Autodesk Inventor part; units mm, degrees
ref_plane "工作平面1" through (65, 2, 0) normal (-1, 0, 0) x (0, 0, 1)
ref_plane "YZ Plane" through (0, 0, 0) normal (1, 0, 0) x (0, 1, 0)
ref_plane "XZ Plane" through (0, 0, 0) normal (0, 1, 0) x (-1, 0, 0)
sketch "草圖1" plane through (0, 0, 0) normal (0, 0, 1) x (1, 0, 0)
  line L0 (0, 0) -> (-7.8042, 0) construction
  line L1 (0, 0) -> (0, -16.694) construction
  line L2 (0, 2) -> (0, 13)
  line L3 (310, 145) -> (310, 102)
  line L4 (130, 19.7875) -> (130, 13) construction
  line L5 (128, 0) -> (2, 0)
  line L6 (310, 145) -> (368, 145)
  line L7 (375, 138) -> (375, 109)
  line L8 (368, 102) -> (310, 102)
  line L9 (332, 127.5) -> (354, 127.5)
  arc A0 (354, 119.5) -> (354, 127.5) centre (354, 123.5) ccw
  line L10 (354, 119.5) -> (332, 119.5)
  arc A1 (332, 127.5) -> (332, 119.5) centre (332, 123.5) ccw
  arc A2 (10.0615, 42.1637) -> (0, 28) centre (15, 28) ccw
  line L11 (10.0615, 42.1637) -> (303.401, 144.4425)
  line L12 (306.6934, 145) -> (310, 145)
  line L13 (310, 102) -> (305, 102)
  line L14 (286.6386, 106.4667) -> (135.4256, 28.6799)
  arc A3 (375, 138) -> (368, 145) centre (368, 138) ccw
  arc A4 (368, 102) -> (375, 109) centre (368, 109) ccw
  arc A5 (302.6723, 103.1075) -> (305, 102) centre (305, 105) ccw
  arc A6 (302.6723, 103.1075) -> (286.6386, 106.4667) centre (292.5854, 94.9066) ccw
  arc A7 (306.6934, 145) -> (303.401, 144.4425) centre (306.6934, 135) ccw
  arc A8 (135.4256, 28.6799) -> (131.466, 25) centre (140, 19.7875) ccw
  line L15 (0, 25) -> (2, 25)
  line L16 (2, 25) -> (2, 13)
  line L17 (2, 13) -> (0, 13)
  line L18 (0, 13) -> (0, 25) construction
  line L19 (65, 0) -> (65, 25) construction
  line L20 (131.466, 25) -> (128, 25)
  line L21 (128, 25) -> (128, 13)
  line L22 (128, 13) -> (130, 13)
  line L23 (130, 13) -> (130, 19.7875) construction
  arc A9 (0, 2) -> (2, 0) centre (2, 2) ccw
  arc A10 (128, 0) -> (130, 2) centre (128, 2) ccw
  line L24 (0, 13) -> (0, 25) construction
  line L25 (0, 25) -> (0, 28)
  line L26 (130, 19.7875) -> (130, 25) construction
  line L27 (130, 13) -> (130, 2)
  line L28 (123.9345, 45) -> (99.3585, 45)
  line L29 (157.566, 75) -> (173.8509, 75)
  line L30 (97.7123, 54.7212) -> (154.2737, 74.4425)
  line L31 (175.452, 68.3877) -> (135.3705, 47.769)
  arc A11 (175.452, 68.3877) -> (173.8509, 75) centre (173.8509, 71.5) ccw
  arc A12 (97.7123, 54.7212) -> (99.3585, 45) centre (99.3585, 50) ccw
  arc A13 (123.9345, 45) -> (135.3705, 47.769) centre (123.9345, 70) ccw
  arc A14 (157.566, 75) -> (154.2737, 74.4425) centre (157.566, 65) ccw
  line L32 (189.9693, 86.8885) -> (229.5263, 100.6808)
  line L33 (231.0996, 97.0139) -> (206.0106, 84.1076)
  line L34 (201.4362, 83) -> (190.6278, 83)
  arc A15 (231.0996, 97.0139) -> (229.5263, 100.6808) centre (230.1847, 98.7923) ccw
  arc A16 (201.4362, 83) -> (206.0106, 84.1076) centre (201.4362, 93) ccw
  arc A17 (189.9693, 86.8885) -> (190.6278, 83) centre (190.6278, 85) ccw
  arc A18 (131.466, 25) -> (130, 19.7875) centre (140, 19.7875) ccw construction
  line L35 (68, 25) -> (68, 17)
  arc A19 (62, 17) -> (68, 17) centre (65, 17) ccw
  line L36 (62, 17) -> (62, 25)
  arc A20 (68, 25) -> (62, 25) centre (65, 25) ccw
  point P0 (130, 0)
  point P1 (375, 145)
  point P2 (375, 102)
  point P3 (130, 25.8889)
  point P4 (305, 145)
  point P5 (305, 102)
  point P6 (305, 115.9121)
  point P7 (0, 10.2)
  point P8 (130, 28)
  point P9 (130, 10.2)
  dimension "d0" = 130
  dimension "d1" = 145
  dimension "d2" = 43
  dimension "d3" = 65
  dimension "d4" = 8
  dimension "d5" = 30
  dimension "d7" = 18
  dimension "d8" = 310
  dimension "d17" = 21.5
  dimension "d20" = 15
  dimension "d21" = 28
  dimension "d23" = 5
  dimension "d24" = 7
  dimension "d26" = 3
  dimension "d29" = 13
  dimension "d30" = 5
  dimension "d31" = 10
  dimension "d32" = 10
  dimension "d33" = 8
  dimension "d39" = 12
  dimension "d40" = 2
  dimension "d41" = 13
  dimension "d42" = 2
  dimension "d45" = 45
  dimension "d46" = 17
  dimension "d47" = 17
  dimension "d48" = 30
  dimension "d49" = 3.5
  dimension "d50" = 5
  dimension "d51" = 25
  dimension "d52" = 10
  dimension "d53" = 8
  dimension "d54" = 2
  dimension "d55" = 10
  dimension "d56" = 2
  dimension "d57" = 19.7875
  dimension "d60" = 6
  dimension "d61" = 8
  dimension "d63" = 17
extrude "擠出1" add sketch "草圖1" along normal blind 2.5
bend part "折彎零件1" radius 0.5 angle 80 line through (310, 145, 0) along (0, -1, 0) centre toward (0, 0, -1) moving side (1, 0, 0) both sides no
ref_plane "工作平面1" through (65, 2, 0) normal (-1, 0, 0) x (0, 0, 1)
properties part number "0 零件" material "不鏽鋼SUS-HL(砂紋)"
Source: CAD feature listing. Evaluate the final solid. Frame: model axes, mm. A direction names the side the tool comes from. Coordinates: 2 decimals unless noted, no trailing zeros. Order: outer loops, then holes, each group sorted by start corner. A loop starts at its lowest first (then second) coordinate and runs counter-clockwise, first axis right, second up. Notation, with made-up numbers: M -15,39 L 28,39 A27 ccw 28,66 Z; hole C 13.5,-37.75 d3. An arc over 180 degrees is marked long. Write each question's results on one line, items separated by ' | '. Start each with the question number.
1. Pin query (flat end, axial travel): pin 1 (0.8 mm diameter, centred on y = 22.5, z = 2, fed in from -X); pin 2 (1.6 mm diameter, centred on x = 1, z = 1, fed in from +Y); pin 3 (19.5 mm diameter, centred on x = 316.5, z = -36, fed in from -Y). Return the tip coordinate at first contact, or that it passes through.
2. Section D-D, the plane x = 87.5. Return the cut outline in (y, z), then the cut area to 3 significant figures.
3. Section B-B, the plane z = -30. Return the cut outline in (x, y), then the cut area to 4 significant figures.
4. Section A-A, the plane x = 196.5. Return the cut outline in (y, z), then the cut area to 3 significant figures.
5. Section C-C, the plane z = -9.5. Return the cut outline in (x, y), then the cut area to 3 significant figures.
6. Reachability of faces 4 (the face through (218.73, 90.65, 1.23)), 5 (the face through (143, 51, 0)), 6 (the face through (317, 119.5, -32)) from +Z, -Z, +X, -X, +Y, -Y: full face, straight path, thin tool, end or side. Return the list, or none.
7. Draft query along Y for faces 1 (the face through (3, 37, 1)), 2 (the face through (155.69, 58.22, 1.23)), 3 (the face through (143, 51, 2.5)). Return one class per face: +Y half, -Y half, draft (parallel to the pull), parting line (faces both ways), or undercut.
8. Material intervals for L1, parallel to Z at x = 226, y = 77; L2, parallel to X at y = 111, z = -54.5; L3, parallel to X at y = 110, z = -57, sorted ascending.
Solution:
1) pin 1: x = 2 | pin 2: y = 35.12 | pin 3: y = 102
2) outline: M 0,0 L 69.16,0 L 69.16,2.5 L 0,2.5 Z | area: 173 mm²
3) outline: M 315.71,102 L 318.25,102 L 318.25,119.5 L 315.71,119.5 Z; M 315.71,127.5 L 318.25,127.5 L 318.25,145 L 315.71,145 Z | area: 88.85 mm²
4) outline: M 60.1,0 L 83,0 L 83,2.5 L 60.1,2.5 Z; M 89.17,0 L 107.17,0 L 107.17,2.5 L 89.17,2.5 Z | area: 102 mm²
5) outline: M 312.09,102 L 314.63,102 L 314.63,145 L 312.09,145 Z | area: 109 mm²
6) face 4: +Z, -Z | face 5: -Z, -X, +Y, -Y | face 6: +X, -X
7) face 1: +Y half | face 2: undercut | face 3: draft
8) L1: 0 to 2.5 | L2: 320.03 to 322.57 | L3: 320.47 to 323.01
